Study the drawing (mm; zero at the part's minimum x, y, z) and answer. Give positions to 0.01 mm unless a question says otherwise; leave off trailing zeros. Order: outer loops, then holes, each group sorted by start corner. A loop starts at its lowest first (then second) coordinate and runs counter-clockwise, first axis right, second up. Notation, with made-up numbers: (46, -9) -> (95, -9) arc R20 cw to (95, 14) -> close; hole circle Ø9 at (81, 43.25). An arc over 180 degrees is marked (long way). Use a Markdown table: item, result. Add a question column.
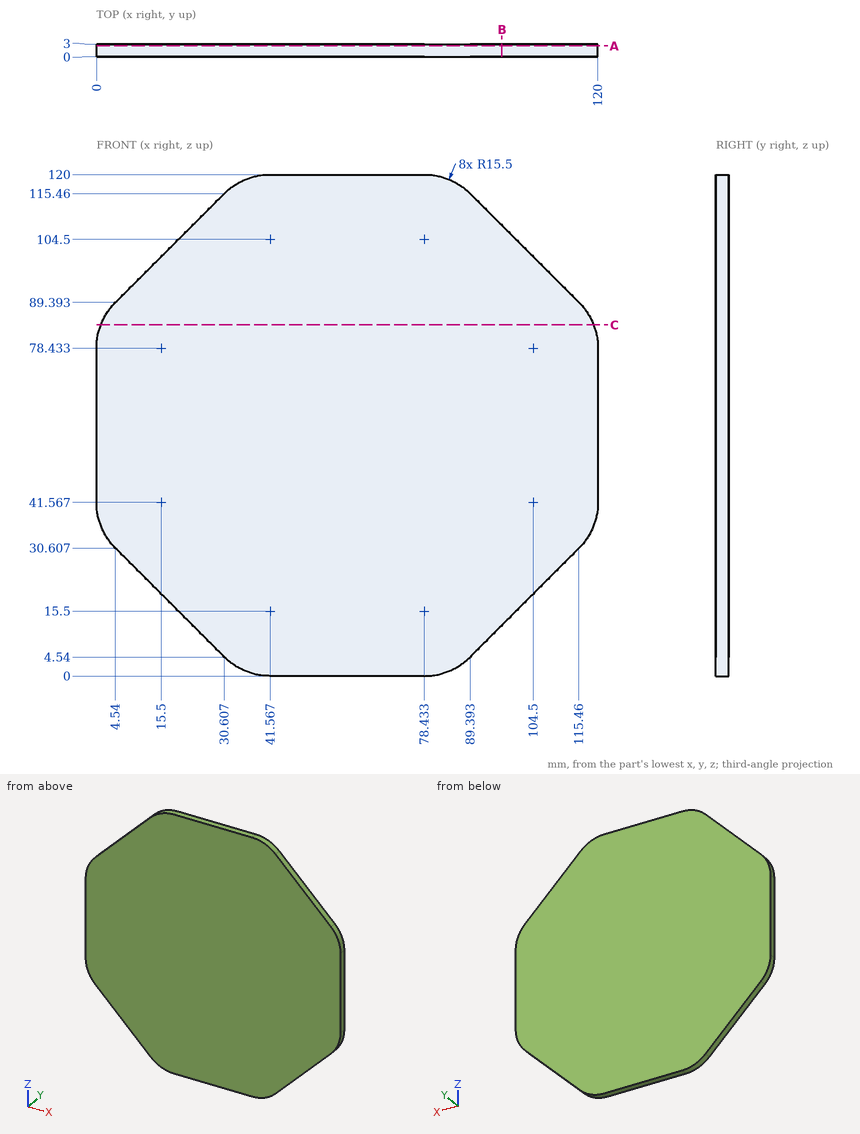
1) The part is cut by section A-A, the plane y = 2.55. Determine the outline of the cut face in (x, z), then the cut area to 3 significant figures.
2) Straight lines are drawn through the part: line 1 (X direction, y = 0.3, z = 81.5); line 2 (X direction, y = 0.6, z = 33) (1 decimal); line 3 (Z direction, x = 88.5, y = 0.45) (1 decimal). For each, find the intervals that lie inside material, in ascending order.
3) The part is cut by section B-B, the plane x = 97. Determine the outline of the cut face in (y, z), then the cut area to 3 significant figures.
4) The part is cut by section C-C, the plane z = 84. Determine the outline of the cut face in (x, y) (1 decimal).
5) A flat-ended cylindrical pin translates along its axis: pin 1 (12 mm diameter, centred on x = 34.5, z = 72.5, fed in from -Y). Find the tip coordinate at first contact, or state that the pin passes through.
A:
| question | item | result |
|---|---|---|
| 1 | outline | (0, 41.57) arc R15.5 ccw to (4.54, 30.61) -> (30.61, 4.54) arc R15.5 ccw to (41.57, 0) -> (78.43, 0) arc R15.5 ccw to (89.39, 4.54) -> (115.46, 30.61) arc R15.5 ccw to (120, 41.57) -> (120, 78.43) arc R15.5 ccw to (115.46, 89.39) -> (89.39, 115.46) arc R15.5 ccw to (78.43, 120) -> (41.57, 120) arc R15.5 ccw to (30.61, 115.46) -> (4.54, 89.39) arc R15.5 ccw to (0, 78.43) -> close |
| 1 | area | 11,900 mm^2 |
| 2 | line 1 | 0.31 to 119.69 |
| 2 | line 2 | 2.6 to 117.4 |
| 2 | line 3 | 3.7 to 116.3 |
| 3 | outline | (0, 12.15) -> (3, 12.15) -> (3, 107.85) -> (0, 107.85) -> close |
| 3 | area | 287 mm^2 |
| 4 | outline | (1, 0) -> (119, 0) -> (119, 3) -> (1, 3) -> close |
| 5 | pin 1 | y = 0 |
